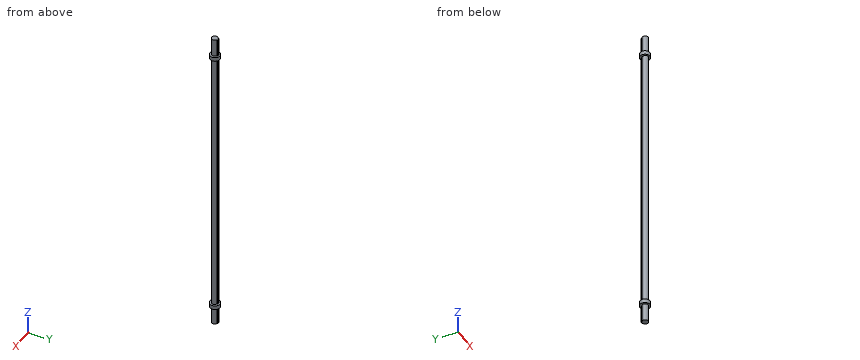
from build123d import *

# Parameters (mm, degrees)
BOSS_EXTRUDE1_DEPTH = 800
SKETCH2_R           = 25
BOSS_EXTRUDE2_DEPTH = 20


with BuildPart() as part:
    # Sketch1 → Boss-Extrude1 (new, symmetric)
    with BuildSketch(Plane.XY):
        with BuildLine():
            Line((-5, 12.492135624), (-5, 16.65))
            Line((-5, 16.65), (5, 16.65))
            Line((5, 16.65), (5, 12.492135624))
            ThreePointArc((5, 12.492135624), (0, -16.65), (-5, 12.492135624))
        make_face()
    extrude(amount=BOSS_EXTRUDE1_DEPTH, both=True)

    # Sketch2 → Boss-Extrude2 (add)
    with BuildSketch(Plane.XY.offset(710)):
        Circle(SKETCH2_R)
    boss_extrude2 = extrude(amount=-BOSS_EXTRUDE2_DEPTH)

    # Mirror1: Boss-Extrude2 across plane
    add(boss_extrude2.mirror(Plane.XY))


solid = part.part
Read the model definition and answer for the solid it produces. Units are mm, in the model's axes. Round coordinates to 2 decimals unless told otherwise and drop trailing zeros. Loops run counter-clockwise (first coordinate to the right, second up) from the corner with the lowest first, then second, coordinate; pieces in that order, holes last.
Q1. Each of these flat-tipped pins is pushed along its axis until it touches: pin 1 (12 mm diameter, centred on x = 13, z = -31, fed in from +Y); pin 2 (11 mm diameter, centred on x = -2, z = 6, fed in from +Y); pin 3 (1 mm diameter, centred on x = 7, z = 50.5, fed in from +Y). Where does it stop, or does it pass through?
Q2. Section B-B on z = 205 is taken. Write down the section's boundary in (x, y), and give its area (3 significant figures).
Q3. Section A-A on y = 0 is taken. Write down the section's boundary in (x, z), and give its area (3 significant figures).
Q4. Consider probe 1 along Z at (x, y) = (16, -8.5); probe 2 along X at (y, z) = (14, 360); probe 3 along X at (y, z) = (-12.5, -526). Determine where each line is inside the solid, lowest interval first.
Output:
1. pin 1: stops at y = 11.62
1. pin 2: stops at y = 16.65
1. pin 3: stops at y = 11.87
2. outline: (-5, 12.49) arc R15 ccw (long way) to (5, 12.49) - (5, 16.65) - (-5, 16.65) - close
2. area: 743 mm2
3. outline: (-25, -710) - (-14.91, -710) - (-14.91, -800) - (14.91, -800) - (14.91, -710) - (25, -710) - (25, -690) - (14.91, -690) - (14.91, 690) - (25, 690) - (25, 710) - (14.91, 710) - (14.91, 800) - (-14.91, 800) - (-14.91, 710) - (-25, 710) - (-25, 690) - (-14.91, 690) - (-14.91, -690) - (-25, -690) - close
3. area: 48,500 mm2
4. probe 1: z = -710 to -690, 690 to 710
4. probe 2: x = -5 to 5
4. probe 3: x = -10.36 to 10.36
